Source: CAD feature listing. Evaluate the final solid. Frame: model axes, mm. Face numbers are marked on the shaded views. A direction names the side the tool comes from. Round coordinates to 2 decimals unless told otherwise and drop trailing zeros. Write each loop counter-clockwise with the first axis right and the second up, starting at its lowest first coordinate (ties: lowest second). Pieces come first, ordered by that corner, then holes.
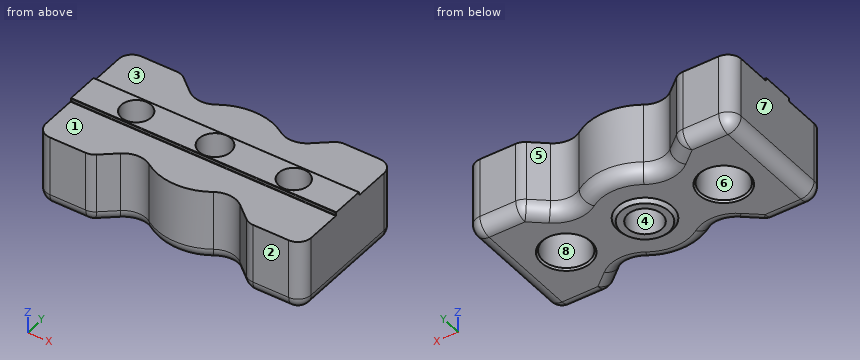
Autodesk Inventor part; units mm, degrees
ref_plane "YZ Plane" through (0, 0, 0) normal (1, 0, 0) x (0, 1, 0)
ref_plane "XZ Plane" through (0, 0, 0) normal (0, 1, 0) x (-1, 0, 0)
ref_plane "XY Plane" through (0, 0, 0) normal (0, 0, 1) x (1, 0, 0)
sketch "Sketch1" plane through (0, 0, 0) normal (0, 0, 1) x (1, 0, 0)
  line L0 (-40, 19.775) -> (40, 19.775)
  line L1 (40, 19.775) -> (40, -19.775)
  line L2 (40, -19.775) -> (-40, -19.775)
  line L3 (-40, -19.775) -> (-40, 19.775)
  line L4 (-40, 19.775) -> (40, -19.775) construction
  line L5 (40, 19.775) -> (-40, -19.775) construction
  line L6 (40, -5) -> (-40, -5)
  line L7 (-40, -5) -> (-40, 5)
  line L8 (-40, 5) -> (40, 5)
  line L9 (40, 5) -> (40, -5)
  line L10 (40, -5) -> (-40, 5) construction
  line L11 (-40, -5) -> (40, 5) construction
  line L12 (23.75, 0) -> (-23.75, 0)
  circle A0 centre (-23.75, 0) radius 4.5
  circle A1 centre (23.75, 0) radius 4.5
  circle A2 centre (0, 0) radius 8
  point P0 (40, 5)
  point P1 (-40, -5)
  point P2 (40, -5)
  point P3 (-6.245, -5)
  point P4 (6.245, -5)
  point P5 (6.245, 5)
  point P6 (-6.245, 5)
  dimension "d0" = 80
  dimension "d1" = 39.55
  dimension "d3" = 10
  dimension "d9" = 80
  dimension "d10" = 47.5
  dimension "d11" = 9
  dimension "d12" = 9
  dimension "d15" = 16
  dimension "d42" = 19.775
  dimension "d43" = 0
extrude "Extrusion1" add sketch "Sketch1" along normal blind 1 contours L8 A2 L6 L3 | L1 L6 A2 L8 | L8 A2 L12 | A2 L12 L6
extrude "Extrusion2" add sketch "Sketch1" against normal blind 6
fillet "Fillet1" radius 0.2 4 edges at (0, 5, 0) (0, 5, 1) (0, -5, 1) (0, -5, 0)
sketch "Sketch2" plane through (0, 0, -6) normal (0, 0, -1) x (-1, 0, 0)
  circle A0 centre (23.75, 0) radius 4.5
  circle A1 centre (-23.75, 0) radius 4.5
  circle A2 centre (23.75, 0) radius 7
  circle A3 centre (-23.75, 0) radius 7
  line L0 (-40, -19.775) -> (40, -19.775)
  line L1 (-40, 19.775) -> (-40, -19.775)
  line L2 (40, 19.775) -> (-40, 19.775)
  line L3 (40, -19.775) -> (40, 19.775)
  point P0 (0, 0)
  dimension "d16" = 14
  dimension "d17" = 14
extrude "Extrusion3" add sketch "Sketch2" along normal blind 16 contours L1 L2 L3 L0
sketch "Sketch3" plane through (0, 0, -22) normal (0, 0, -1) x (-1, 0, 0)
  circle A0 centre (0, 0) radius 5.15
  dimension "d21" = 10.3
extrude "Extrusion4" cut sketch "Sketch3" against normal blind 10
sketch "Sketch4" plane through (0, 0, -22) normal (0, 0, -1) x (-1, 0, 0)
  circle A0 centre (0, 0) radius 5.15
  circle A1 centre (0, 0) radius 7.25
  dimension "d24" = 14.5
extrude "Extrusion5" add sketch "Sketch4" along normal blind 1
chamfer "Chamfer1" distance 1 distance2 1 1 edges at (7.25, 0, -22) measured on face at (-0.2913, -15.5824, -22)
sketch "Sketch5" plane through (0, 0, -12) normal (0, 0, -1) x (-1, 0, 0)
  circle A0 centre (0, 0) radius 4.8
  dimension "d30" = 9.6
extrude "Extrusion6" cut sketch "Sketch5" against normal blind 20
sketch "Sketch6" plane through (0, 0, -22) normal (0, 0, -1) x (-1, 0, 0)
  circle A0 centre (0, 0) radius 17.5
  circle A1 centre (23.75, 0) radius 7
  circle A2 centre (-23.75, 0) radius 7
  line L0 (40, -19.775) -> (40, 19.775)
  line L1 (40, 19.775) -> (-40, 19.775)
  line L2 (-40, 19.775) -> (-40, -19.775)
  line L3 (-40, -19.775) -> (40, -19.775)
  circle A3 centre (0, 0) radius 8.25
  line L4 (-23.75, 0) -> (-23.75, 19.775)
  line L5 (13.4485, 11.1977) -> (23.75, 19.775)
  line L6 (-40, 19.775) -> (40, 19.775)
  line L7 (-23.75, 19.775) -> (-13.4485, 11.1977)
  dimension "d33" = 35
extrude "Extrusion7" cut sketch "Sketch6" against normal through all contours A0 L7 L1 L5
mirror "Mirror1" about plane through (0, 0, 0) normal (0, 1, 0) of "Extrusion7"
fillet "Fillet3" radius 7 4 edges at (13.4485, 11.1977, -11) (-13.4485, 11.1977, -11) (13.4485, -11.1977, -11) (-13.4485, -11.1977, -11)
fillet "Fillet4" radius 4 8 edges at (23.75, -19.775, -11) (40, -19.775, -11) (40, 19.775, -11) (23.75, 19.775, -11) (-23.75, 19.775, -11) (-40, 19.775, -11) (-40, -19.775, -11) (-23.75, -19.775, -11)
fillet "Fillet5" radius 4 24 edges at (38.8284, 18.6034, -22) (40, 0, -22) (38.8284, -18.6034, -22) (30.5986, -19.775, -22) (23.8363, -19.5364, -22) (20.3404, -16.9361, -22) (13.9404, -13.4128, -22) (0, -17.5, -22) (-13.9404, -13.4128, -22) (-20.3404, -16.9361, -22) (-23.8363, -19.5364, -22) (-30.5986, -19.775, -22) (-38.8284, -18.6034, -22) (-40, 0, -22) (-38.8284, 18.6034, -22) (-30.5986, 19.775, -22) (-23.8363, 19.5364, -22) (-20.3404, 16.9361, -22) (-13.9404, 13.4128, -22) (0, 17.5, -22) (13.9404, 13.4128, -22) (20.3404, 16.9361, -22) (23.8363, 19.5364, -22) (30.5986, 19.775, -22)
chamfer "Chamfer2" distance 0.5 angle 45 2 edges at (-16.75, 0, -22) (30.75, 0, -22)
equation "\"d9\" = d0"
properties part number "Base_Mount_Pedals"
1) Reachability of the marked faces 1, 2, 3 and 4 from +Z, -Z, +X, -X, +Y, -Y: full face, straight path, thin tool, end or side. Return the list, or none.
Taken from the geometry:
face 1: +Z, +X, -X, -Y
face 2: +Z, -Z, +X, -X, -Y
face 3: +Z, +X, -X, +Y
face 4: -Z
2) Pull-direction query (Y, two-part tool) for the marked faces 5, 6, 7 and 8; classes: released by +Y, released by -Y, zero draft, split by the parting line, or undercut.
Taken from the geometry:
face 5: released by +Y
face 6: undercut
face 7: zero draft
face 8: undercut
3) Section query B-B on y = 0. State how many separate pieces and enclosed holes the cut face has, then the cut area to 3 significant figures.
Taken from the geometry:
separate pieces: 4
enclosed holes: 0
area: 1,040 mm2
4) Section query A-A on z = -7.75. Return the cut outline in (x, y) (3 decimals).
Taken from the geometry:
outline: (-40, -15.775) arc R4 ccw to (-36, -19.775) - (-25.197, -19.775) arc R4 ccw to (-22.638, -18.849) - (-18.043, -15.023) arc R7 cw to (-9.689, -14.573) arc R17.5 ccw to (9.689, -14.573) arc R7 cw to (18.043, -15.023) - (22.638, -18.849) arc R4 ccw to (25.197, -19.775) - (36, -19.775) arc R4 ccw to (40, -15.775) - (40, 15.775) arc R4 ccw to (36, 19.775) - (25.197, 19.775) arc R4 ccw to (22.638, 18.849) - (18.043, 15.023) arc R7 cw to (9.689, 14.573) arc R17.5 ccw to (-9.689, 14.573) arc R7 cw to (-18.043, 15.023) - (-22.638, 18.849) arc R4 ccw to (-25.197, 19.775) - (-36, 19.775) arc R4 ccw to (-40, 15.775) - close; hole circle Ø14 at (-23.75, 0); hole circle Ø9.6 at (0, 0); hole circle Ø14 at (23.75, 0)
5) Section query C-C on z = -14.5. Return the cut outline in (x, y) (3 decimals).
Taken from the geometry:
outline: (-40, -15.775) arc R4 ccw to (-36, -19.775) - (-25.197, -19.775) arc R4 ccw to (-22.638, -18.849) - (-18.043, -15.023) arc R7 cw to (-9.689, -14.573) arc R17.5 ccw to (9.689, -14.573) arc R7 cw to (18.043, -15.023) - (22.638, -18.849) arc R4 ccw to (25.197, -19.775) - (36, -19.775) arc R4 ccw to (40, -15.775) - (40, 15.775) arc R4 ccw to (36, 19.775) - (25.197, 19.775) arc R4 ccw to (22.638, 18.849) - (18.043, 15.023) arc R7 cw to (9.689, 14.573) arc R17.5 ccw to (-9.689, 14.573) arc R7 cw to (-18.043, 15.023) - (-22.638, 18.849) arc R4 ccw to (-25.197, 19.775) - (-36, 19.775) arc R4 ccw to (-40, 15.775) - close; hole circle Ø14 at (-23.75, 0); hole circle Ø10.3 at (0, 0); hole circle Ø14 at (23.75, 0)
6) Material intervals for line 1 (X direction, y = -3.5, z = -18.5); line 2 (X direction, y = 0.5, z = -11); line 3 (X direction, y = -14, z = -13.5), sorted ascending.
Taken from the geometry:
line 1: x = -39.97 to -29.81, -17.69 to -3.78, 3.78 to 17.69, 29.81 to 39.97
line 2: x = -40 to -30.73, -16.77 to -4.77, 4.77 to 16.77, 30.73 to 40
line 3: x = -40 to -16.39, -10.73 to 10.73, 16.39 to 40
7) Contact query for flat-ended pins moving along their axis: P1, Ø12, axis at x = 0, y = 0, coming from the -Z side; P2, Ø2, axis at x = 25, y = 12.5, coming from the -Z side; P3, Ø2, axis at x = -22, y = 13, coming from the +Z side; P4, Ø5.5, axis at x = -23.75, y = 0, coming from the -Z side. Output: stop coordinate, or through.
Taken from the geometry:
P1: stops at z = -23
P2: stops at z = -22
P3: stops at z = 0
P4: passes through
